```python
from build123d import *

# Parameters (mm, degrees)
SKETCH1_W            = 12.15
SKETCH1_H            = 10.15
EXTRUDE2_DEPTH       = 9
SKETCH11_R           = 1.95
EXTRUDE5_DEPTH       = 0.6
EXTRUDE6_DEPTH       = 9.27
EXTRUDE7_DEPTH       = 15
SKETCH14_R           = 2.5
EXTRUDE8_DEPTH       = 1.5
SKETCH16_W           = 0.3
SKETCH16_H           = 1.5
EXTRUDE10_DEPTH      = 2
FILLET1_R            = 0.3
FILLET1_OF_MIRROR1_R = 0.3
FILLET2_R            = 0.5
FILLET3_R            = 0.3
SKETCH17_R           = 0.5
EXTRUDE11_DEPTH      = 7.75


with BuildPart() as part:
    # Sketch1 → Extrude2 (new body)
    with BuildSketch(Plane.XY):
        Rectangle(SKETCH1_W, SKETCH1_H)
    extrude(amount=-EXTRUDE2_DEPTH)

    # Sketch11 → Extrude5 (add)
    with BuildSketch(Plane.XY):
        Circle(SKETCH11_R)
    extrude(amount=EXTRUDE5_DEPTH)

    # Sketch12 → Extrude6 (add)
    with BuildSketch(Plane.XY.offset(0.6)):
        with BuildLine():
            Line((-1.17260394, 0.975), (1.17260394, 0.975))
            ThreePointArc((1.17260394, 0.975), (0, -1.525), (-1.17260394, 0.975))
        make_face()
    extrude(amount=EXTRUDE6_DEPTH)

    # Sketch13 → Extrude7 (add)
    with BuildSketch(Plane(origin=(0, 0, -9), x_dir=(-1, 0, 0), z_dir=(0, 0, -1))):
        with BuildLine():
            Line((-3.494281042, 5), (3.494281042, 5))
            ThreePointArc((3.494281042, 5), (6.1, 0), (3.494281042, -5))
            Line((3.494281042, -5), (-3.494281042, -5))
            ThreePointArc((-3.494281042, -5), (-6.1, 0), (-3.494281042, 5))
        make_face()
    extrude(amount=EXTRUDE7_DEPTH)

    # Sketch14 → Extrude8 (add)
    with BuildSketch(Plane(origin=(0, 0, -24), x_dir=(-1, 0, 0), z_dir=(0, 0, -1))):
        Circle(SKETCH14_R)
    extrude(amount=EXTRUDE8_DEPTH)

    # Sketch16 → Extrude10 (add)
    with BuildSketch(Plane(origin=(0, 0, -24), x_dir=(-1, 0, 0), z_dir=(0, 0, -1))):
        with Locations((3.5, 0)):
            Rectangle(SKETCH16_W, SKETCH16_H)
    extrude10 = extrude(amount=EXTRUDE10_DEPTH)

    # Fillet1
    fillet1_edges = [part.edges().sort_by_distance(p)[0] for p in [
        (-3.5, -0.75, -26),
        (-3.5, 0.75, -26),
    ]]
    fillet(fillet1_edges, radius=FILLET1_R)

    # Mirror1: Extrude10 across plane
    add(extrude10.mirror(Plane(origin=(0, 0, 0), x_dir=(0, 0, 1), z_dir=(1, 0, 0))))

    # Fillet1 of Mirror1
    fillet1_of_mirror1_edges = [part.edges().sort_by_distance(p)[0] for p in [
        (3.5, -0.75, -26),
        (3.5, 0.75, -26),
    ]]
    fillet(fillet1_of_mirror1_edges, radius=FILLET1_OF_MIRROR1_R)

    # Fillet2
    fillet2_edges = [part.edges().sort_by_distance(p)[0] for p in [
        (-6.075, 5.075, -4.5),
        (6.075, 5.075, -4.5),
        (6.075, -5.075, -4.5),
        (-6.075, -5.075, -4.5),
    ]]
    fillet(fillet2_edges, radius=FILLET2_R)

    # Fillet3
    fillet3_edges = [part.edges().sort_by_distance(p)[0] for p in [
        (2.5, 0, -25.5),
    ]]
    fillet(fillet3_edges, radius=FILLET3_R)

    # Sketch17 → Extrude11 (add)
    with BuildSketch(Plane(origin=(0, 0, -25.5), x_dir=(-1, 0, 0), z_dir=(0, 0, -1))):
        Circle(SKETCH17_R)
    extrude(amount=EXTRUDE11_DEPTH)


solid = part.part
```
Part model, mm, in its own coordinate system. A direction names the side the tool comes from. Round coordinates to 2 decimals unless told otherwise and drop trailing zeros. Write each loop counter-clockwise with the first axis right and the second up, starting at its lowest first coordinate (ties: lowest second). Pieces come first, ordered by that corner, then holes. Notation, with made-up numbers: (12.25, -28.75) -> (37.25, -28.75) arc R32 ccw to (37.25, 0.25) -> close; hole circle Ø7 at (25, 1.25). An arc over 180 degrees is marked (long way). Return JSON: item names as keys, results as strings. Group by question number.
Q1. Probe L1, parallel to Z at x = -4.5, y = 2.75; L2, parallel to Y at x = 2.25, z = -15; L3, parallel to X at y = -2, z = -25. List the from-to ranges inside material, lowest first. Write a range as [from, to].
Q2. Pin check, flat tips, straight feed: pin 1 (3 mm diameter, centred on y = -2.5, z = -4.5, fed in from -X) (3 decimals); pin 2 (5 mm diameter, centred on x = 3.5, y = -2.5, fed in from -Z); pin 3 (4 mm diameter, centred on x = 0, z = -23.5, fed in from -Y). Stop position of each tip, or through.
Q3. Saw through at C-C on z = -10. Write the cut outline in (x, y).
Q4. Which spindle directions (+Z, -Z, +X, -X, +Y, -Y) get a long thin tool onto all of the face, cutting with end or side? Do faces 4 (the flat face through (0, -5, -16)), 5 (the cylindrical face through (0.108, -0.488, -29.321)), 6 (the flat face through (-3.35, 0, -25)), 7 (the cylindrical face through (-6.1, 0.1, -16.4)). Say none if no direction does.
Q5. Saw through at D-D on x = -4.75. Write the cut outline in (y, z) (3 decimals).
Q6. Saw through at A-A on x = 0. Write the cut outline in (y, z) (3 decimals), plus the area to 3 significant figures.
Q7. Mould opens along X. For faces 1 (the cylindrical face through (6.1, -0.1, -16.4)), 2 (the cylindrical face through (0.048, -1.524, 5.17)), 3 (the flat face through (0, 1, -25.5)) say: pulls with the +X half, pulls with the -X half, needs draft (parallel to the pull), parting line crosses it, or undercut.
Answer:
{
 "1": {"L1": "[-24, 0]", "L2": "[-5, 5]", "L3": "[-1.5, 1.5]"},
 "2": {"pin 1": "x = -6.075", "pin 2": "z = -26", "pin 3": "y = -5"},
 "3": {"outline": "(-3.49, -5) -> (3.49, -5) arc R6.1 ccw to (3.49, 5) -> (-3.49, 5) arc R6.1 ccw to start"},
 "4": {"face 4": "-Z, +X, -X, -Y", "face 5": "-Z", "face 6": "-Z, +Y, -Y", "face 7": "-Z, -X"},
 "5": {"outline": "(-5.075, -9) -> (-3.827, -9) -> (-3.827, -24) -> (3.827, -24) -> (3.827, -9) -> (5.075, -9) -> (5.075, 0) -> (-5.075, 0) -> close"},
 "6": {"outline": "(-5.075, -9) -> (-5, -9) -> (-5, -24) -> (-2.5, -24) -> (-2.5, -25.2) arc R0.3 ccw to (-2.2, -25.5) -> (-0.5, -25.5) -> (-0.5, -33.25) -> (0.5, -33.25) -> (0.5, -25.5) -> (2.2, -25.5) arc R0.3 ccw to (2.5, -25.2) -> (2.5, -24) -> (5, -24) -> (5, -9) -> (5.075, -9) -> (5.075, 0) -> (1.95, 0) -> (1.95, 0.6) -> (0.975, 0.6) -> (0.975, 9.87) -> (-1.525, 9.87) -> (-1.525, 0.6) -> (-1.95, 0.6) -> (-1.95, 0) -> (-5.075, 0) -> close", "area": "282 mm2"},
 "7": {"face 1": "pulls with the +X half", "face 2": "parting line crosses it", "face 3": "undercut"}
}
